Could you check a few things on this drawing? It's one solid part, dimensions in mm from its lowest x, y, z. Coordinates: 2 decimals unless noted, no trailing zeros. Order: outer loops, then holes, each group sorted by start corner. A loop starts at its lowest first (then second) coordinate and runs counter-clockwise, first axis right, second up. Notation, with made-up numbers: (-6.5, 84) - (52.5, 84) arc R13 ccw to (52.5, 102) - close; hole circle Ø9 at (55.5, 15.25). An arc over 180 degrees is marked (long way). Return JSON: item names as keys, results as strings. Group by question number.
1) If I drill on line 1 along Y through (x, z) = (30.5, 251.5); line 2 along Y through (x, z) = (22, 21.5), over which ranges is the centre line in solid material (lowest first)?
2) Imagine slicing it at A-A (x = 24). Write out the boundary of the cut face in (y, z), and give its area (3 significant figures).
3) If we mould it in two halves opening along Y, with no side actions, what happens to the marked faces 1, 2, 3 and 4? For each: pulls with the +Y half, pulls with the -Y half, needs draft (parallel to the pull), parting line crosses it, or undercut.
4) Imagine slicing it at D-D (z = 326.5). Write out the boundary of the cut face in (x, y).
5) Imagine slicing it at B-B (y = 48.5). Write out the boundary of the cut face in (x, z), and give its area (3 significant figures).
6) Imagine slicing it at C-C (z = 246.5). Write out the boundary of the cut face in (x, y), and give its area (3 significant figures).
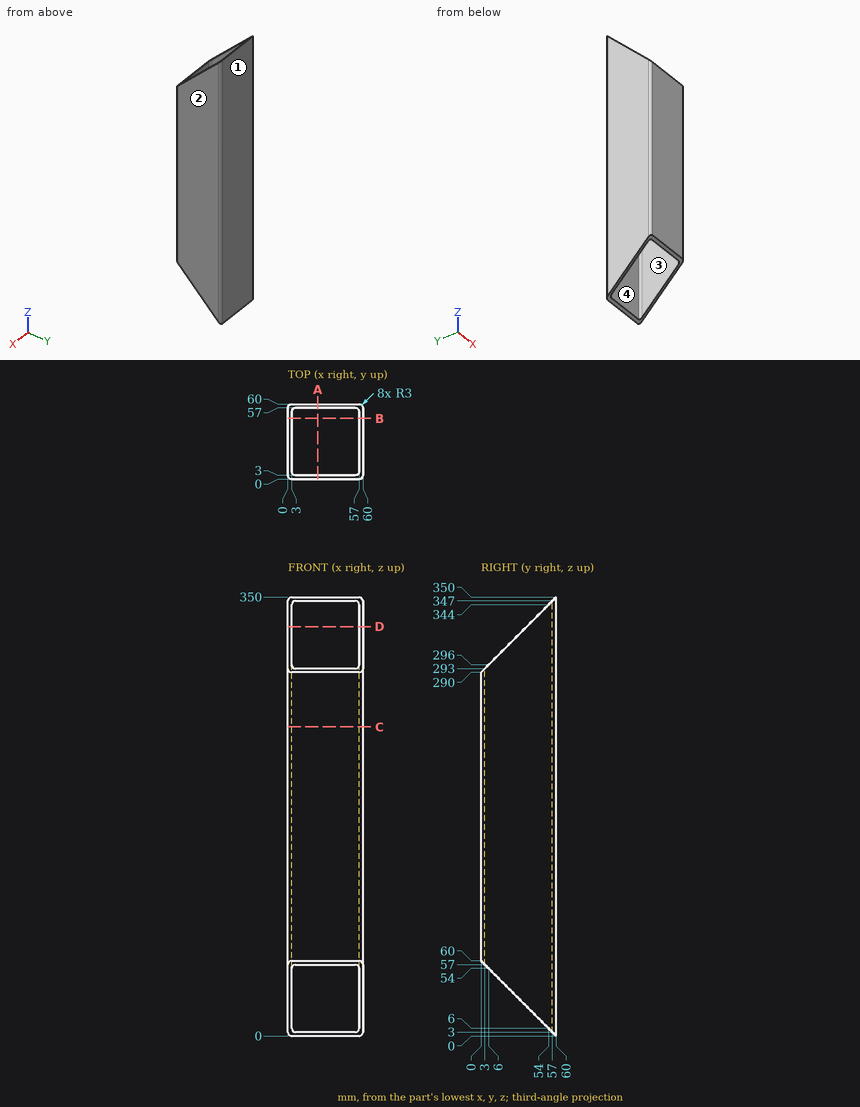
Calculated:
{
 "1": {"line 1": "0 to 3, 57 to 60", "line 2": "57 to 60"},
 "2": {"outline": "(0, 60) - (3, 57) - (3, 293) - (0, 290) - close; (57, 3) - (60, 0) - (60, 350) - (57, 347) - close", "area": "1,740 mm2"},
 "3": {"face 1": "pulls with the +Y half", "face 2": "needs draft", "face 3": "undercut", "face 4": "undercut"},
 "4": {"outline": "(0, 36.5) - (3, 36.5) - (3, 54) arc R3 cw to (6, 57) - (54, 57) arc R3 cw to (57, 54) - (57, 36.5) - (60, 36.5) - (60, 57) arc R3 ccw to (57, 60) - (3, 60) arc R3 ccw to (0, 57) - close"},
 "5": {"outline": "(0, 11.5) - (3, 11.5) - (3, 338.5) - (0, 338.5) - close; (57, 11.5) - (60, 11.5) - (60, 338.5) - (57, 338.5) - close", "area": "1,960 mm2"},
 "6": {"outline": "(0, 3) arc R3 ccw to (3, 0) - (57, 0) arc R3 ccw to (60, 3) - (60, 57) arc R3 ccw to (57, 60) - (3, 60) arc R3 ccw to (0, 57) - close; hole (3, 6) arc R3 ccw to (6, 3) - (54, 3) arc R3 ccw to (57, 6) - (57, 54) arc R3 ccw to (54, 57) - (6, 57) arc R3 ccw to (3, 54) - close", "area": "684 mm2"}
}
